Job drawing, mm, ordinate dimensions from the low corner. One solid piece. A direction names the side the tool comes from. Round coordinates to 2 decimals unless told otherwise and drop trailing zeros. Loops run counter-clockwise (first coordinate to the right, second up) from the corner with the lowest first, then second, coordinate; pieces in that order, holes last.
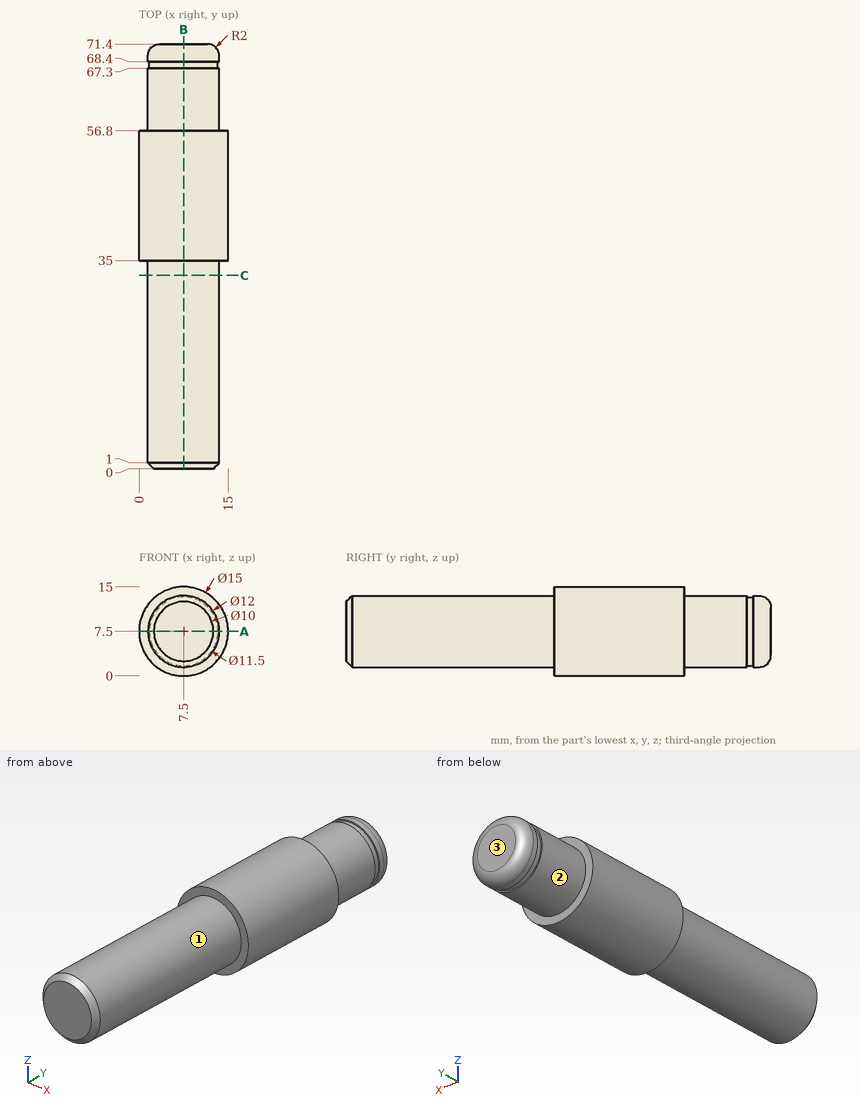
Item 1: Cut at B-B, the plane x = 7.5. Give the cut face in (y, z).
Answers follow:
outline: (0, 2.5) - (1, 1.5) - (35, 1.5) - (35, 0) - (56.8, 0) - (56.8, 1.5) - (67.3, 1.5) - (67.3, 1.75) - (68.4, 1.75) - (68.4, 1.5) - (69.4, 1.5) arc R2 ccw to (71.4, 3.5) - (71.4, 11.5) arc R2 ccw to (69.4, 13.5) - (68.4, 13.5) - (68.4, 13.25) - (67.3, 13.25) - (67.3, 13.5) - (56.8, 13.5) - (56.8, 15) - (35, 15) - (35, 13.5) - (1, 13.5) - (0, 12.5) - close
Item 2: Cut at C-C, the plane y = 32.5. Give the cut face in (x, z), plus the area to 3 significant figures.
Answers follow:
outline: circle Ø12 at (7.5, 7.5)
area: 113 mm2
Item 3: Cut at A-A, the plane z = 7.5. Give the cut face in (x, y), plus the area to 3 significant figures.
Answers follow:
outline: (0, 35) - (1.5, 35) - (1.5, 1) - (2.5, 0) - (12.5, 0) - (13.5, 1) - (13.5, 35) - (15, 35) - (15, 56.8) - (13.5, 56.8) - (13.5, 67.3) - (13.25, 67.3) - (13.25, 68.4) - (13.5, 68.4) - (13.5, 69.4) arc R2 ccw to (11.5, 71.4) - (3.5, 71.4) arc R2 ccw to (1.5, 69.4) - (1.5, 68.4) - (1.75, 68.4) - (1.75, 67.3) - (1.5, 67.3) - (1.5, 56.8) - (0, 56.8) - close
area: 919 mm2
Item 4: Probe line 1 (Y direction, x = 11, z = 2.5); line 2 (Y direction, x = 12.5, z = 10.5); line 3 (X direction, y = 16.5, z = 7.25). List the from-to ranges inside material, lowest first.
Answers follow:
line 1: y = 35 to 56.8
line 2: y = 0.83 to 67.3, 68.4 to 70.2
line 3: x = 1.51 to 13.49
Item 5: 3-axis set-ups, long thin cutter, end or side, ignore diameter. For the marked faces 1, 2 and 3: which of +Z, -Z, +X, -X, +Y, -Y reach the whole face in a straight line?
Answers follow:
face 1: -Y
face 2: +Y
face 3: +Z, -Z, +X, -X, +Y
Item 6: Flat gauge pins, fed straight in: P1, Ø1, axis at y = 17.5, z = 3, coming from the -X side; P2, Ø5, axis at y = 59.5, z = 4.5, coming from the +X side; P3, Ø2, axis at y = 21.5, z = 8, coming from the -X side. Where does each tip first touch, or does it go through?
Answers follow:
P1: stops at x = 3.03
P2: stops at x = 13.48
P3: stops at x = 1.5
